Source: three-view drawing plus pictorial views. Frame: mm from the lowest corner of the part. A direction names the side the tool comes from. Coordinates: 2 decimals unless noted, no trailing zeros. Write each loop counter-clockwise with the first axis right and the second up, starting at its lowest first coordinate (ties: lowest second). Pieces come first, ordered by that corner, then holes. Notation, with made-up numbers: (-8, 57.25) - (49, 57.25) arc R26 ccw to (49, 80.25) - close; hole circle Ø8 at (-40, -5). An arc over 180 degrees is marked (long way). Put each result on its own line as item: value.
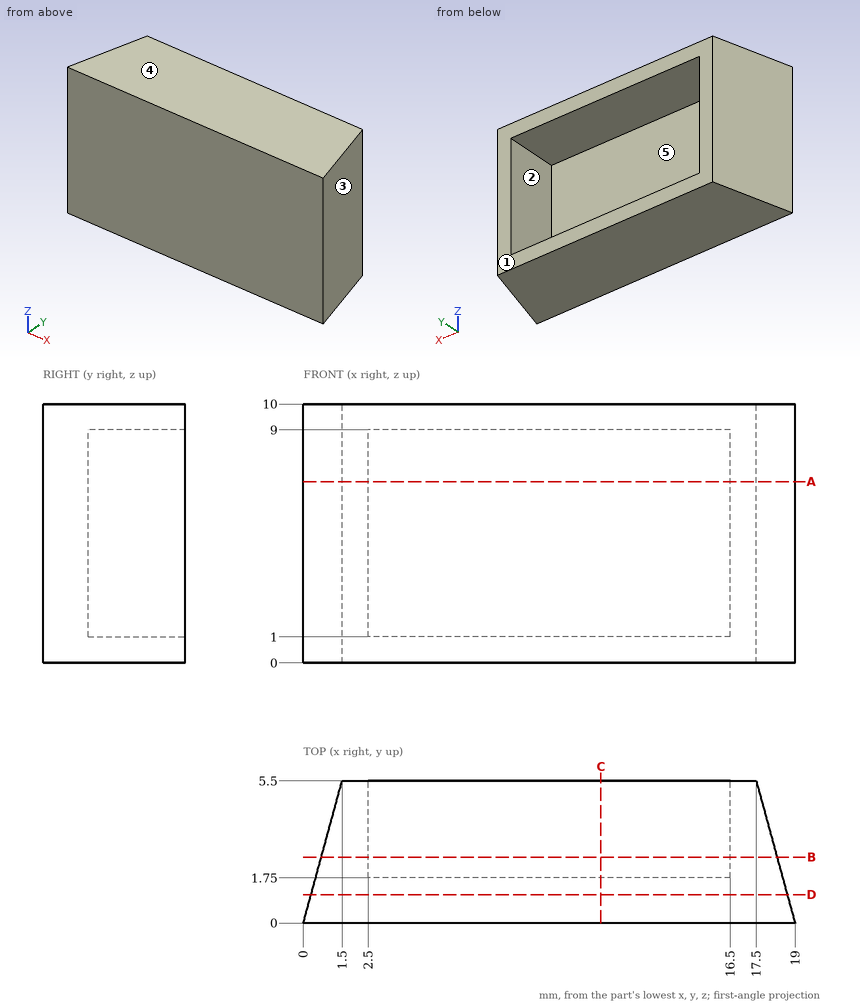
1. Pin query (flat end, axial travel): pin 1 Ø2 at (x, z) = (8.5, 6.5) entering from -Y; pin 2 Ø3 at (y, z) = (4, 7) entering from +X; pin 3 Ø1.1 at (y, z) = (4.5, 6) entering from -X. Return the tip coordinate at first contact, or that it passes through.
Answer below:
pin 1: stops at y = 0
pin 2: stops at x = 18.32
pin 3: stops at x = 1.08
2. Section query B-B (y = 2.55). Return loops of the section in (x, z).
Answer below:
outline: (0.7, 0) - (18.3, 0) - (18.3, 10) - (0.7, 10) - close; hole (2.5, 1) - (16.5, 1) - (16.5, 9) - (2.5, 9) - close
3. Section query A-A (z = 7). Return loops of the section in (x, y), then the cut area to 4 significant figures.
Answer below:
outline: (0, 0) - (19, 0) - (17.5, 5.5) - (16.5, 5.5) - (16.5, 1.75) - (2.5, 1.75) - (2.5, 5.5) - (1.5, 5.5) - close
area: 43.75 mm²
4. Mould query, pull axis X, two halves, no side actions, for the marked faces 3, 4 and 5. Classes: +X half, -X half, draft (parallel to the pull), parting line (faces both ways), or undercut.
Answer below:
face 3: +X half
face 4: draft
face 5: undercut
5. Ray query, probe 1 along Z at (x, y) = (16, 5.1); probe 2 along Y at (x, z) = (14.5, 6.75); probe 3 along X at (y, z) = (4.8, 7.75). Return the intervals inside material, ascending. Write a range as from..to.
Answer below:
probe 1: z = 0..1, 9..10
probe 2: y = 0..1.75
probe 3: x = 1.31..2.5, 16.5..17.69
6. Set-up query: the marked faces 1 and 2. Return all of +Z, -Z, +X, -X, +Y, -Y with unobstructed straight access to the full face (end or side cutting, diameter ignored); none if empty.
Answer below:
face 1: +Z, -Z, +X, -X, +Y
face 2: +Y
7. Section query D-D (y = 1.1). Return loops of the section in (x, z).
Answer below:
outline: (0.3, 0) - (18.7, 0) - (18.7, 10) - (0.3, 10) - close
8. Section query C-C (x = 11.5). Return loops of the section in (y, z).
Answer below:
outline: (0, 0) - (5.5, 0) - (5.5, 1) - (1.75, 1) - (1.75, 9) - (5.5, 9) - (5.5, 10) - (0, 10) - close
